Autodesk Inventor part; units mm, degrees
ref_plane "YZ Plane" through (0, 0, 0) normal (1, 0, 0) x (0, 1, 0)
ref_plane "XZ Plane" through (0, 0, 0) normal (0, 1, 0) x (-1, 0, 0)
ref_plane "XY Plane" through (0, 0, 0) normal (0, 0, 1) x (1, 0, 0)
sketch "adapter-hole-geometry" plane through (0, 0, 0) normal (0, 0, 1) x (1, 0, 0)
  line L0 (15.875, -11.43) -> (-15.875, -11.43) construction
  line L1 (-15.875, -11.43) -> (-15.875, 11.43) construction
  line L2 (-15.875, 11.43) -> (15.875, 11.43) construction
  line L3 (15.875, 11.43) -> (15.875, -11.43) construction
  line L4 (15.875, -11.43) -> (-15.875, 11.43) construction
  line L5 (-15.875, -11.43) -> (15.875, 11.43) construction
  line L6 (11.43, -15.875) -> (-11.43, -15.875) construction
  line L7 (-11.43, -15.875) -> (-11.43, 15.875) construction
  line L8 (-11.43, 15.875) -> (11.43, 15.875) construction
  line L9 (11.43, 15.875) -> (11.43, -15.875) construction
  line L10 (11.43, -15.875) -> (-11.43, 15.875) construction
  line L11 (-11.43, -15.875) -> (11.43, 15.875) construction
  line L12 (0, -8.4414) -> (8.4414, 0) construction
  line L13 (8.4414, 0) -> (0, 8.4414) construction
  line L14 (0, 8.4414) -> (-8.4414, 0) construction
  line L15 (-8.4414, 0) -> (0, -8.4414) construction
  line L16 (-5.969, -5.969) -> (5.969, 5.969) construction
  line L17 (5.969, -5.969) -> (-5.969, 5.969) construction
  line L18 (-8.4414, -8.4414) -> (8.4414, -8.4414) construction
  line L19 (8.4414, -8.4414) -> (8.4414, 8.4414) construction
  line L20 (8.4414, 8.4414) -> (-8.4414, 8.4414) construction
  line L21 (-8.4414, 8.4414) -> (-8.4414, -8.4414) construction
  line L22 (-8.4414, -8.4414) -> (8.4414, 8.4414) construction
  line L23 (8.4414, -8.4414) -> (-8.4414, 8.4414) construction
  point P0 (0, 0)
  point P1 (0, 8.4414)
  point P2 (8.4414, 0)
  dimension "d29" = 31.75
  dimension "d30" = 22.86
  dimension "d31" = 22.86
  dimension "d32" = 31.75
  dimension "d33" = 11.938
  dimension "d34" = 11.938
  dimension "d42" = 16.8829
  dimension "d43" = 16.8829
  dimension "d58" = 4.445
  dimension "d59" = 7.4336
  dimension "d60" = 5.969
  dimension "d61" = 5.969
  dimension "d62" = 4.445
  dimension "d63" = 7.4336
  dimension "d64" = 9.906
  dimension "d65" = 9.906
  dimension "d66" = 15.875
  dimension "d67" = 5.969
  dimension "d68" = 21.844
  dimension "d69" = 21.844
sketch "Sketch1" plane through (0, 0, 0) normal (0, 0, 1) x (1, 0, 0)
  line L0 (19.05, -19.05) -> (-19.05, -19.05)
  line L1 (-19.05, -19.05) -> (-19.05, 19.05)
  line L2 (-19.05, 19.05) -> (19.05, 19.05)
  line L3 (19.05, 19.05) -> (19.05, -19.05)
  line L4 (19.05, -19.05) -> (-19.05, 19.05) construction
  line L5 (-19.05, -19.05) -> (19.05, 19.05) construction
  point P0 (0, 0)
  dimension "d0" = 38.1
  dimension "d1" = 38.1
extrude "Extrusion1" add sketch "Sketch1" along normal blind 0.7937
sketch "Sketch4" plane through (0, 0, 0.7937) normal (0, 0, 1) x (1, 0, 0)
  line L0 (-19.05, -19.05) -> (19.05, -19.05) construction
  line L1 (19.05, -19.05) -> (19.05, 19.05) construction
  line L2 (19.05, 19.05) -> (-19.05, 19.05) construction
  line L3 (-19.05, 19.05) -> (-19.05, -19.05) construction
  point P0 (0, 0)
  point P1 (-15.875, 11.43)
  point P2 (-15.875, 0)
  point P3 (-15.875, -11.43)
  point P4 (15.875, -11.43)
  point P5 (15.875, 0)
  point P6 (15.875, 11.43)
  point P7 (0, 8.4414)
  point P8 (-8.4414, 0)
  point P9 (0, -8.4414)
  point P10 (8.4414, 0)
  dimension "d44" = 3.175
  dimension "d45" = 3.175
  dimension "d46" = 7.62
  dimension "d47" = 3.175
  dimension "d48" = 7.62
  dimension "d49" = 3.175
  dimension "d50" = 7.62
hole "Hole3" at (-15.875, 11.43, 0.7937) at (-15.875, 0, 0.7937) at (-15.875, -11.43, 0.7937) at (15.875, -11.43, 0.7937) at (15.875, 0, 0.7937) at (15.875, 11.43, 0.7937) at (0, 8.4414, 0.7937) at (-8.4414, 0, 0.7937) at (0, -8.4414, 0.7937) at (8.4414, 0, 0.7937) direction (0, 0, -1) diameter 3.7973 end through all
properties part number "goniometer_stage_shim_v1" material "Stainless Steel AISI 304"
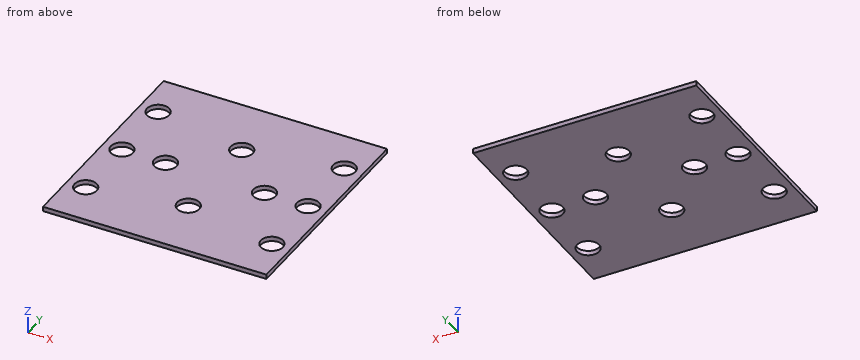
Check sheet for the modelled part. Datum: model origin and axes. Units: mm. Round coordinates to 2 decimals unless told otherwise and drop trailing zeros. Order: outer loops, then holes, each group sorted by start corner. A loop starts at its lowest first (then second) coordinate and runs counter-clockwise, first axis right, second up. Notation, with made-up numbers: (65.5, 20) -> (124.5, 20) arc R13 cw to (124.5, 41) -> close; hole circle Ø2 at (23, 70). An arc over 180 degrees is marked (long way). One line per item, written item: value. Start each with the question number.
Q1. Cross-section at B-B (y = -11.43). Record the boundary of the cut face in (x, z), and give its area (3 significant figures).
Q2. Cross-section at A-A (y = 0). Record the boundary of the cut face in (x, z).
Q3. Cross-section at D-D (y = 8.5). Record the boundary of the cut face in (x, z).
Q4. Gauge pin test, flat end, axial feed: pin 1 Ø3 at (x, y) = (0, -8.44) entering from +Z. Record the tip position at first contact, or that the pin passes through.
Q5. Cross-section at C-C (x = 0). Record the boundary of the cut face in (y, z), and give its area (3 significant figures).
Q6. Thickness scan on line 1 (X direction, y = -11.43, z = 0.5); line 2 (X direction, y = 0, z = 0.45); line 3 (Y direction, x = -16, z = 0.1). Record the ranges inside material, lowest first.
Completed:
1. outline: (-19.05, 0) -> (-17.77, 0) -> (-17.77, 0.79) -> (-19.05, 0.79) -> close; (-13.98, 0) -> (13.98, 0) -> (13.98, 0.79) -> (-13.98, 0.79) -> close; (17.77, 0) -> (19.05, 0) -> (19.05, 0.79) -> (17.77, 0.79) -> close
1. area: 24.2 mm²
2. outline: (-19.05, 0) -> (-17.77, 0) -> (-17.77, 0.79) -> (-19.05, 0.79) -> close; (-13.98, 0) -> (-10.34, 0) -> (-10.34, 0.79) -> (-13.98, 0.79) -> close; (-6.54, 0) -> (6.54, 0) -> (6.54, 0.79) -> (-6.54, 0.79) -> close; (10.34, 0) -> (13.98, 0) -> (13.98, 0.79) -> (10.34, 0.79) -> close; (17.77, 0) -> (19.05, 0) -> (19.05, 0.79) -> (17.77, 0.79) -> close
3. outline: (-19.05, 0) -> (-1.9, 0) -> (-1.9, 0.79) -> (-19.05, 0.79) -> close; (1.9, 0) -> (19.05, 0) -> (19.05, 0.79) -> (1.9, 0.79) -> close
4. pin 1: passes through
5. outline: (-19.05, 0) -> (-10.34, 0) -> (-10.34, 0.79) -> (-19.05, 0.79) -> close; (-6.54, 0) -> (6.54, 0) -> (6.54, 0.79) -> (-6.54, 0.79) -> close; (10.34, 0) -> (19.05, 0) -> (19.05, 0.79) -> (10.34, 0.79) -> close
5. area: 24.2 mm²
6. line 1: x = -19.05 to -17.77, -13.98 to 13.98, 17.77 to 19.05
6. line 2: x = -19.05 to -17.77, -13.98 to -10.34, -6.54 to 6.54, 10.34 to 13.98, 17.77 to 19.05
6. line 3: y = -19.05 to -13.32, -9.54 to -1.89, 1.89 to 9.54, 13.32 to 19.05
